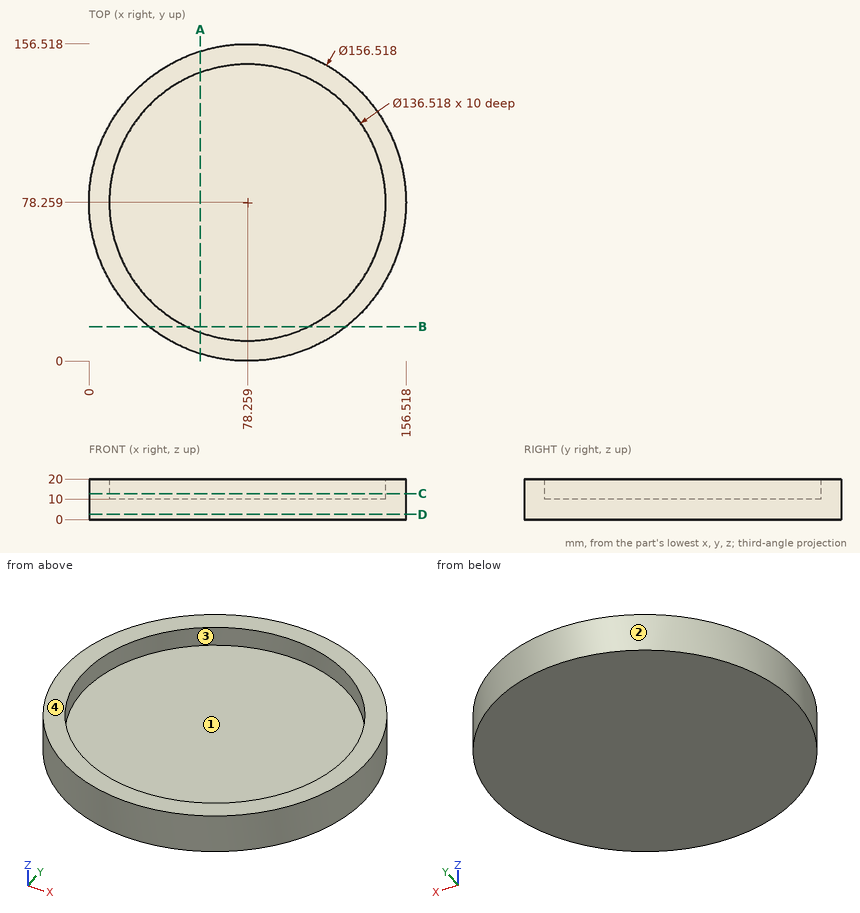
Answer from the drawing. Dimensions are ordinates in mm from the lowest x, y and z of the part. Coordinates: 2 decimals unless noted, no trailing zeros. Order: outer loops, then holes, each group sorted by start corner. A loop starts at its lowest first (then second) coordinate and runs counter-clockwise, first axis right, second up. Notation, with made-up numbers: M 46.5,-12 L 70.5,-12 A9 ccw 70.5,2 Z; hole C -5.75,-34 d11. An arc over 180 degrees is marked long. Put each result on its own line as item: value. Start each with the question number.
Item 1: Section B-B, the plane y = 17 is taken. Determine the outline of the cut face in (x, z), plus the area to 3 significant figures.
Item 2: Section A-A, the plane x = 55 is taken. Determine the outline of the cut face in (y, z) (1 decimal), plus the area to 3 significant figures.
Item 3: Section C-C, the plane z = 12.75 is taken. Determine the outline of the cut face in (x, y), plus the area to 3 significant figures.
Item 4: The mould has two halves that part along Y. Classify the marked faces 1, 2, 3 and 4: +Y half, -Y half, draft (parallel to the pull), parting line (faces both ways), or undercut.
Item 5: Consider probe 1 along Z at (x, y) = (59, 124.5); probe 2 along X at (y, z) = (50, 13.75) (1 decimal); probe 3 along Y at (x, z) = (56, 10.25) (1 decimal). Determine where each line is inside the solid, lowest interval first. Write a range as [from, to].
Item 6: Section D-D, the plane z = 2.5 is taken. Determine the outline of the cut face in (x, y).
Item 7: Given pin 1 Ø1 at (x, z) = (108, 3.5) entering from +Y; pin 2 Ø10 at (y, z) = (77, 12.5) entering from -X; pin 3 Ø1.5 at (y, z) = (65, 10) entering from +X; pin 4 Ø5 at (x, z) = (135, 14.5) entering from +Y, each flat-ended and moving along its own axis, determine where each tip first touches the part or whether it passes through.
Computed:
1. outline: M 29.56,0 L 126.96,0 L 126.96,20 L 108.37,20 L 108.37,10 L 48.15,10 L 48.15,20 L 29.56,20 Z
1. area: 1,350 mm2
2. outline: M 3.5,0 L 153,0 L 153,20 L 142.4,20 L 142.4,10 L 14.1,10 L 14.1,20 L 3.5,20 Z
2. area: 1,710 mm2
3. outline: C 78.26,78.26 d156.52; hole C 78.26,78.26 d136.52
3. area: 4,600 mm2
4. face 1: undercut
4. face 2: parting line
4. face 3: undercut
4. face 4: draft
5. probe 1: z = [0, 10]
5. probe 2: x = [5.3, 16.1], [140.4, 151.2]
5. probe 3: y = [3.2, 13.7], [142.8, 153.3]
6. outline: C 78.26,78.26 d156.52
7. pin 1: stops at y = 150.85
7. pin 2: stops at x = 0
7. pin 3: stops at x = 155.51
7. pin 4: stops at y = 134.67
